Drawing for the job (mm, zero at the part's lowest x, y, z). A direction names the side the tool comes from. Coordinates: 2 decimals unless noted, no trailing zeros. Order: outer loops, then holes, each group sorted by start corner. A loop starts at its lowest first (then second) coordinate and runs counter-clockwise, first axis right, second up. Notation, with made-up numbers: (-23.75, 40) -> (-17.75, 40) arc R13 ccw to (-17.75, 62) -> close; hole circle Ø6 at (45, -22). An arc over 180 degrees is marked (long way). Write each question's results on one line, items separated by ' | '.
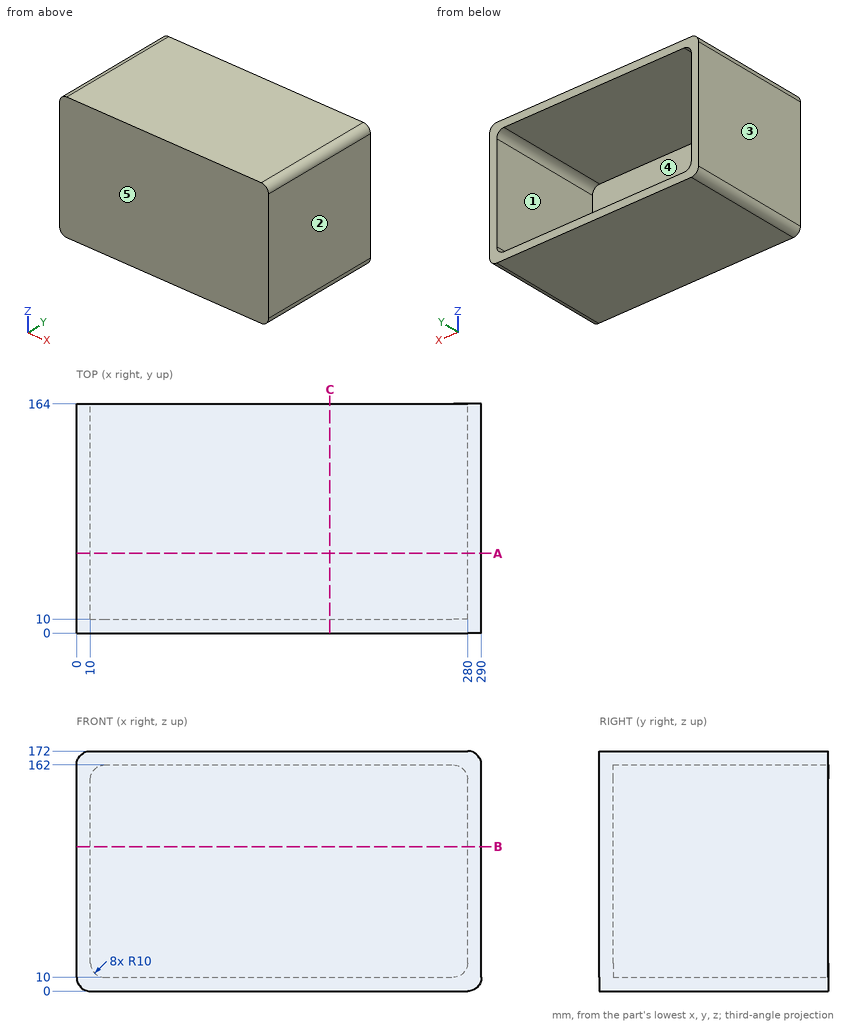
Item 1: Tool access for the marked faces 4 and 5: list every direction of +Z, -Z, +X, -X, +Y, -Y with a clear straight run to the whole face (end or side of a thin tool).
Answer:
face 4: +Y | face 5: +Z, -Z, +X, -X, -Y
Item 2: Slice it at A-A, the plane y = 57. List the corners of the cut face in (x, z).
Answer:
outline: (0, 10) arc R10 ccw to (10, 0) -> (280, 0) arc R10 ccw to (290, 10) -> (290, 162) arc R10 ccw to (280, 172) -> (10, 172) arc R10 ccw to (0, 162) -> close; hole (10, 20) arc R10 ccw to (20, 10) -> (270, 10) arc R10 ccw to (280, 20) -> (280, 152) arc R10 ccw to (270, 162) -> (20, 162) arc R10 ccw to (10, 152) -> close
Item 3: Slice it at C-C, the plane x = 181.5. List the corners of the cut face in (y, z).
Answer:
outline: (0, 0) -> (164, 0) -> (164, 10) -> (10, 10) -> (10, 162) -> (164, 162) -> (164, 172) -> (0, 172) -> close
Item 4: Pull direction X, two halves, no side cores. Call the marked faces 1, 2 and 3: released by +X, released by -X, zero draft, split by the parting line, or undercut.
Answer:
face 1: undercut | face 2: released by +X | face 3: released by -X
Item 5: Slice it at B-B, the plane z = 103.5. List the corners of the cut face in (x, y).
Answer:
outline: (0, 0) -> (290, 0) -> (290, 164) -> (280, 164) -> (280, 10) -> (10, 10) -> (10, 164) -> (0, 164) -> close
Item 6: Drill centre lines: line 1 (X direction, y = 145.5, z = 72.5); line 2 (Z direction, x = 21.5, y = 137); line 3 (Y direction, x = 44, z = 30). Where is each one in solid material? Low to high. Write a range as from..to.
Answer:
line 1: x = 0..10, 280..290 | line 2: z = 0..10, 162..172 | line 3: y = 0..10
